from build123d import *

# Parameters (mm, degrees)
SKETCH1_W           = 25.4
SKETCH1_H           = 101.6
SKETCH1_R           = 8.255
BOSS_EXTRUDE1_DEPTH = 2.54
SKETCH3_W           = 2.54
SKETCH3_H           = 25.4
BOSS_EXTRUDE2_DEPTH = 12.7
SKETCH2_R           = 1.016
CUT_EXTRUDE3_DEPTH  = 12.7
FILLET1_R           = 6.35
SKETCH5_R           = 2.032
CUT_EXTRUDE4_DEPTH  = 1.27
SKETCH6_W           = 2.54
SKETCH6_H           = 12.7
CUT_EXTRUDE5_DEPTH  = 91.696141042


with BuildPart() as part:
    # Sketch1 → Boss-Extrude1 (new body)
    with BuildSketch(Plane(origin=(0, 0, 0), x_dir=(1, 0, 0), z_dir=(0, 1, 0))):
        with Locations((0, 38.1)):
            Rectangle(SKETCH1_W, SKETCH1_H)
        with Locations(Location((0, 0, 0), (0, 0, 270))):
            Circle(SKETCH1_R, mode=Mode.SUBTRACT)
    extrude(amount=BOSS_EXTRUDE1_DEPTH)

    # Sketch3 → Boss-Extrude2 (add)
    with BuildSketch(Plane.XZ):
        with Locations((-11.43, -76.2)):
            Rectangle(SKETCH3_W, SKETCH3_H)
        with Locations((11.43, -76.2)):
            Rectangle(SKETCH3_W, SKETCH3_H)
    extrude(amount=BOSS_EXTRUDE2_DEPTH)

    # Sketch2 → Cut-Extrude3 (cut)
    with BuildSketch(Plane(origin=(0, 2.54, 0), x_dir=(1, 0, 0), z_dir=(0, 1, 0))):
        with Locations(Location((-8.000000002, 22.098, 0), (0, 0, 270))):
            Circle(SKETCH2_R)
        with Locations(Location((8.000000002, 22.098, 0), (0, 0, 90))):
            Circle(SKETCH2_R)
        with Locations(Location((-8.000000002, -7.874, 0), (0, 0, 270))):
            Circle(SKETCH2_R)
        with Locations(Location((8.000000002, -7.874, 0), (0, 0, 90))):
            Circle(SKETCH2_R)
    extrude(amount=-CUT_EXTRUDE3_DEPTH, mode=Mode.SUBTRACT)

    # Fillet1
    fillet1_edges = [part.edges().sort_by_distance(p)[0] for p in [
        (12.7, 1.27, 12.7),
        (-12.7, 1.27, 12.7),
        (12.7, -5.08, -88.9),
        (-12.7, -5.08, -88.9),
    ]]
    fillet(fillet1_edges, radius=FILLET1_R)

    # Sketch5 → Cut-Extrude4 (cut)
    with BuildSketch(Plane.XZ):
        with Locations(Location((-8.000000002, -22.098, 0), (0, 0, 270))):
            Circle(SKETCH5_R)
        with Locations(Location((-8.000000002, 7.874, 0), (0, 0, 270))):
            Circle(SKETCH5_R)
        with Locations(Location((8.000000002, -22.098, 0), (0, 0, 270))):
            Circle(SKETCH5_R)
        with Locations(Location((8.000000002, 7.874, 0), (0, 0, 270))):
            Circle(SKETCH5_R)
    extrude(amount=-CUT_EXTRUDE4_DEPTH, mode=Mode.SUBTRACT)

    # Sketch6 → Cut-Extrude5 (cut, through all)
    with BuildSketch(Plane.XZ):
        with Locations((11.43, -50.8)):
            Rectangle(SKETCH6_W, SKETCH6_H)
        with Locations((-11.43, -50.8)):
            Rectangle(SKETCH6_W, SKETCH6_H)
    extrude(amount=-CUT_EXTRUDE5_DEPTH, mode=Mode.SUBTRACT)


solid = part.part
Could you check a few things on this model? Use its own coordinates, in mm. A direction names the side the tool comes from. Coordinates: 2 decimals unless noted, no trailing zeros. Loops run counter-clockwise (first coordinate to the right, second up) from the corner with the lowest first, then second, coordinate; pieces in that order, holes last.
1. For P1, Ø3.5, axis at x = -7, z = 7.5, coming from the -Y side; P2, Ø2, axis at y = 2, z = -48.5, coming from the +X side; P3, Ø1.3, axis at x = 11, y = -7, coming from the +Z side, each with a flat end and sliding along its axis, tell me the tip position at first contact or that it passes through.
2. Imagine slicing it at D-D (z = -42). Please give me the cut outline in (x, y), and give its area (3 significant figures).
3. For faces 5 (the face through (-11, 1, -57.15)), 6 (the face through (11, -6, -63.5)), 7 (the face through (0, 2.54, -39)), 8 (the face through (10.16, 1, -51)), 9 (the face through (10.16, -6, -76)), which set-ups out of +Z, -Z, +X, -X, +Y, -Y let a thin tool reach every point of the face, with its end or its side?
4. Imagine slicing it at B-B (y = -4.5). Please give me the cut outline in (x, z).
5. Imagine slicing it at A-A (x = 0). Please give me the cut outline in (y, z) (3 decimals), and give its area (3 significant figures).
6. I need wall thicknesses on L1, parallel to X at y = -5.25, z = -64.5; L2, parallel to Y at x = -7.5, z = -61; L3, parallel to Z at x = 5, y = 0.75. Which ranges of each line are inside material? Lowest first, please.
7. Imagine slicing it at C-C (z = -74). Please give me the cut outline in (x, y).
8. We'd pull the mould along X, two halves only. Please class faces 1 (the face through (6.76, 0.63, -20.49)), 2 (the face through (12.075, -5.187, -85.297)), 3 (the face through (-12.7, 1, -19)), 4 (the face through (-11, 1, -44.45)): released by +X, released by -X, zero draft, split by the parting line, or undercut.
Computed values:
1. P1: stops at y = 0
1. P2: stops at x = 10.16
1. P3: stops at z = -63.5
2. outline: (-12.7, 0) - (12.7, 0) - (12.7, 2.54) - (-12.7, 2.54) - close
2. area: 64.5 mm2
3. face 5: -X, +Y, -Y
3. face 6: +Z, +X, -X, -Y
3. face 7: +Z, -Z, +X, -X, +Y
3. face 8: +X, +Y, -Y
3. face 9: +Z, -Z, -Y
4. outline: (-12.7, -82.55) arc R6.35 ccw to (-10.16, -87.63) - (-10.16, -63.5) - (-12.7, -63.5) - close; (10.16, -87.63) arc R6.35 ccw to (12.7, -82.55) - (12.7, -63.5) - (10.16, -63.5) - close
5. outline: (0, -88.9) - (2.54, -88.9) - (2.54, -8.255) - (0, -8.255) - close; (0, 8.255) - (2.54, 8.255) - (2.54, 12.7) - (0, 12.7) - close
5. area: 216 mm2
6. L1: x = -12.7 to -10.16, 10.16 to 12.7
6. L2: y = 0 to 2.54
6. L3: z = -88.9 to -6.57, 6.57 to 12.7
7. outline: (-12.7, -12.7) - (-10.16, -12.7) - (-10.16, 0) - (10.16, 0) - (10.16, -12.7) - (12.7, -12.7) - (12.7, 2.54) - (-12.7, 2.54) - close
8. face 1: undercut
8. face 2: released by +X
8. face 3: released by -X
8. face 4: zero draft
